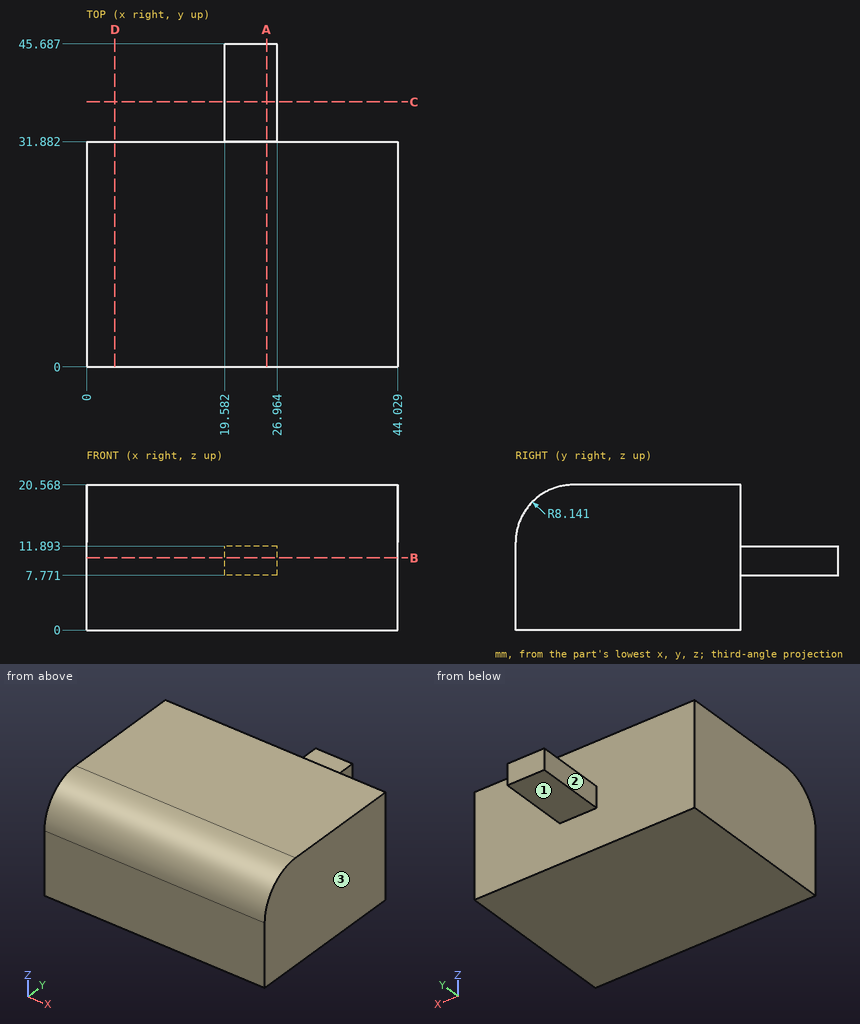
Design review of the part shown in the three views and the two pictorial views. Dimensions are in mm from the part's minimum x, y and z. A direction names the side the tool comes from. Give positions to 0.01 mm unless a question says otherwise; leave off trailing zeros. Write each loop counter-clockwise with the first axis right and the second up, starting at its lowest first coordinate (ties: lowest second). Pieces come first, ordered by that corner, then holes.
Item 1: Insertion check: P1, Ø4.5, axis at y = 39.5, z = 9.5, coming from the +X side; P2, Ø12, axis at x = 17, y = 39, coming from the +Z side; P3, Ø1.2, axis at y = 41.5, z = 10, coming from the -X side; P4, Ø3, axis at y = 35, z = 4.5, coming from the -X side. Each pin has a flat end and moves straight along its axis. Give the tip position at first contact, or say it passes through.
Item 2: Machinability: for the marked faces 1, 2 and 3, which of the approach directions +Z, -Z, +X, -X, +Y, -Y give a long, thin tool a straight path to every point of the face, cutting with its end or side? Answer none if there is none.
Item 3: Wall thickness on probe 1 along Y at (x, z) = (37, 12.25); probe 2 along X at (y, z) = (35, 10.5); probe 3 along Z at (x, y) = (23, 36): over which ranges is each line inside the solid? List them lowest first.
Item 4: Take a section at C-C (y = 37.5). Give the boundary of the cut face in (x, z).
Item 5: Take a section at A-A (x = 25.5). Give the boundary of the cut face in (y, z).
Item 6: Take a section at B-B (z = 10.25). Give the boundary of the cut face in (x, y).
Item 7: Take a section at D-D (x = 4). Give the boundary of the cut face in (y, z).
Established:
1. P1: stops at x = 26.96
1. P2: stops at z = 11.89
1. P3: stops at x = 19.58
1. P4: passes through
2. face 1: -Z, +X, -X, +Y
2. face 2: +Z, -Z, -X, +Y
2. face 3: +Z, -Z, +X, +Y, -Y
3. probe 1: y = 0 to 31.88
3. probe 2: x = 19.58 to 26.96
3. probe 3: z = 7.77 to 11.89
4. outline: (19.58, 7.77) - (26.96, 7.77) - (26.96, 11.89) - (19.58, 11.89) - close
5. outline: (0, 0) - (31.88, 0) - (31.88, 7.77) - (45.69, 7.77) - (45.69, 11.89) - (31.88, 11.89) - (31.88, 20.57) - (8.14, 20.57) arc R8.14 ccw to (0, 12.43) - close
6. outline: (0, 0) - (44.03, 0) - (44.03, 31.88) - (26.96, 31.88) - (26.96, 45.69) - (19.58, 45.69) - (19.58, 31.88) - (0, 31.88) - close
7. outline: (0, 0) - (31.88, 0) - (31.88, 20.57) - (8.14, 20.57) arc R8.14 ccw to (0, 12.43) - close
